```python
from build123d import *

# Parameters (mm, degrees)
SKETCH1_R               = 9.398
BOSS_EXTRUDE1_DEPTH     = 16.2941
SKETCH2_OUTSIDE_W       = 27.032
SKETCH2_OUTSIDE_H       = 27.032
SKETCH2_OUTSIDE_R       = 6.35
CUT_EXTRUDE1_DEPTH      = 7.9375
FILLET1_SIZE            = 2.54
SKETCH3_W               = 19.304
SKETCH3_H               = 2.032
BOSS_EXTRUDE2_DEPTH     = 3.556
CIRPATTERN1_COUNT       = 12
CUT_EXTRUDE2_START      = -9.398
SKETCH5_W               = 10.16
SKETCH5_H               = 0.254
CUT_EXTRUDE2_DEPTH      = 0.254
CIRPATTERN2_COUNT       = 12
CUT_EXTRUDE3_DEPTH      = 25.090427103
CUT_EXTRUDE3_DEPTH_BACK = 25.090427103
SKETCH6_R               = 3.57505


with BuildPart() as part:
    # Sketch1 → Boss-Extrude1 (new body)
    with BuildSketch(Plane.XY):
        Circle(SKETCH1_R)
    extrude(amount=BOSS_EXTRUDE1_DEPTH)

    # Sketch2 outside → Cut-Extrude1 (cut)
    with BuildSketch(Plane.XY.offset(16.2941)):
        Rectangle(SKETCH2_OUTSIDE_W, SKETCH2_OUTSIDE_H)
        Circle(SKETCH2_OUTSIDE_R, mode=Mode.SUBTRACT)
    extrude(amount=-CUT_EXTRUDE1_DEPTH, mode=Mode.SUBTRACT)

    # Fillet1
    # a fillet whose section is not a circle: 2.54 mm, written as the material it adds along each edge
    with BuildSketch(Plane(origin=(0, 0, 8.3566), x_dir=(1, 0, 0), z_dir=(0, -1, 0))) as fillet1_piece_1:
        with BuildLine():
            Bezier((6.35 + FILLET1_SIZE, 0), (6.35, 0), (6.35, FILLET1_SIZE), weights=[1, 0.047339252, 1])
            Line((6.35, FILLET1_SIZE), (6.35, 0))
            Line((6.35, 0), (6.35 + FILLET1_SIZE, 0))
        make_face()
    revolve(axis=Axis((0, 0, 8.3566), (0, 0, 1)))

    # Sketch3 → Boss-Extrude2 (add)
    with BuildSketch(Plane(origin=(0, 0, 0), x_dir=(-1, 0, 0), z_dir=(0, 0, -1))):
        Rectangle(SKETCH3_W, SKETCH3_H)
    boss_extrude2 = extrude(amount=BOSS_EXTRUDE2_DEPTH)

    # CirPattern1: Boss-Extrude2 ×12 about axis
    cirpattern1_axis = Axis((0, 0, 0), (0, 0, 1))
    for i in range(1, CIRPATTERN1_COUNT):
        add(boss_extrude2.rotate(cirpattern1_axis, i * 360 / CIRPATTERN1_COUNT))

    # Sketch5 → Cut-Extrude2 (cut)
    with BuildSketch(Plane(origin=(0, 0, 0), x_dir=(0, 0, -1), z_dir=(1, 0, 0)).offset(CUT_EXTRUDE2_START)):
        with Locations((-5.08, 0)):
            Rectangle(SKETCH5_W, SKETCH5_H)
    cut_extrude2 = extrude(amount=CUT_EXTRUDE2_DEPTH, mode=Mode.SUBTRACT)

    # CirPattern2: Cut-Extrude2 ×12 about axis
    cirpattern2_axis = Axis((0, 0, 0), (0, 0, 1))
    for i in range(1, CIRPATTERN2_COUNT):
        add(cut_extrude2.rotate(cirpattern2_axis, i * 360 / CIRPATTERN2_COUNT), mode=Mode.SUBTRACT)

    # Sketch6 → Cut-Extrude3 (cut, two sides: drawn at the far end of the back side and taken through both)
    with BuildSketch(Plane.XY.offset(16.2941).offset(-CUT_EXTRUDE3_DEPTH_BACK)):
        Circle(SKETCH6_R)
    extrude(amount=CUT_EXTRUDE3_DEPTH + CUT_EXTRUDE3_DEPTH_BACK, mode=Mode.SUBTRACT)


solid = part.part
```
Check sheet for the modelled part. Datum: model origin and axes. Units: mm. A direction names the side the tool comes from. Round coordinates to 2 decimals unless told otherwise and drop trailing zeros. Put each result on its own line as item: value.
(1) Go/stop test with flat-tipped pins: pin 1 Ø3 at (x, z) = (2.5, 4.5) entering from -Y; pin 2 Ø4 at (x, z) = (3.5, 13) entering from +Y; pin 3 Ø1.5 at (y, z) = (1.5, 2) entering from +X. Record where each tip stops, or that it passes through.
Values found:
pin 1: stops at y = -9.34
pin 2: stops at y = 6.17
pin 3: stops at x = 9.37
(2) Material ranges on line 1 (Y direction, x = 0, z = 2.5); line 2 (Y direction, x = 0, z = 12.25), recorded low to high.
Values found:
line 1: y = -9.14 to -3.58, 3.58 to 9.14
line 2: y = -6.35 to -3.58, 3.58 to 6.35
(3) Tool access check on faces 1 (the face through (-2.5, 6.36, -1.75)), 2 (the face through (-5, -5, 0)), 3 (the face through (9.086, 2.401, 4.12)). Record the directions out of +Z, -Z, +X, -X, +Y, -Y that give a thin tool (end or side, any length) a straight path to the whole face; none if there is none.
Values found:
face 1: -Z, +Y
face 2: -Z
face 3: +Z, +X, +Y
(4) Mould release check, pull along Y, two halves, no side actions. Record for faces 4 (the face through (5, 5, 0)), 5 (the face through (8.37, 4.81, -1.75)), 6 (the face through (-1.016, 7, -2)), 7 (the face through (-9.086, -2.401, 4.12)): released by +Y, released by -Y, zero draft, split by the parting line, or undercut.
Values found:
face 4: undercut
face 5: released by +Y
face 6: zero draft
face 7: released by -Y
